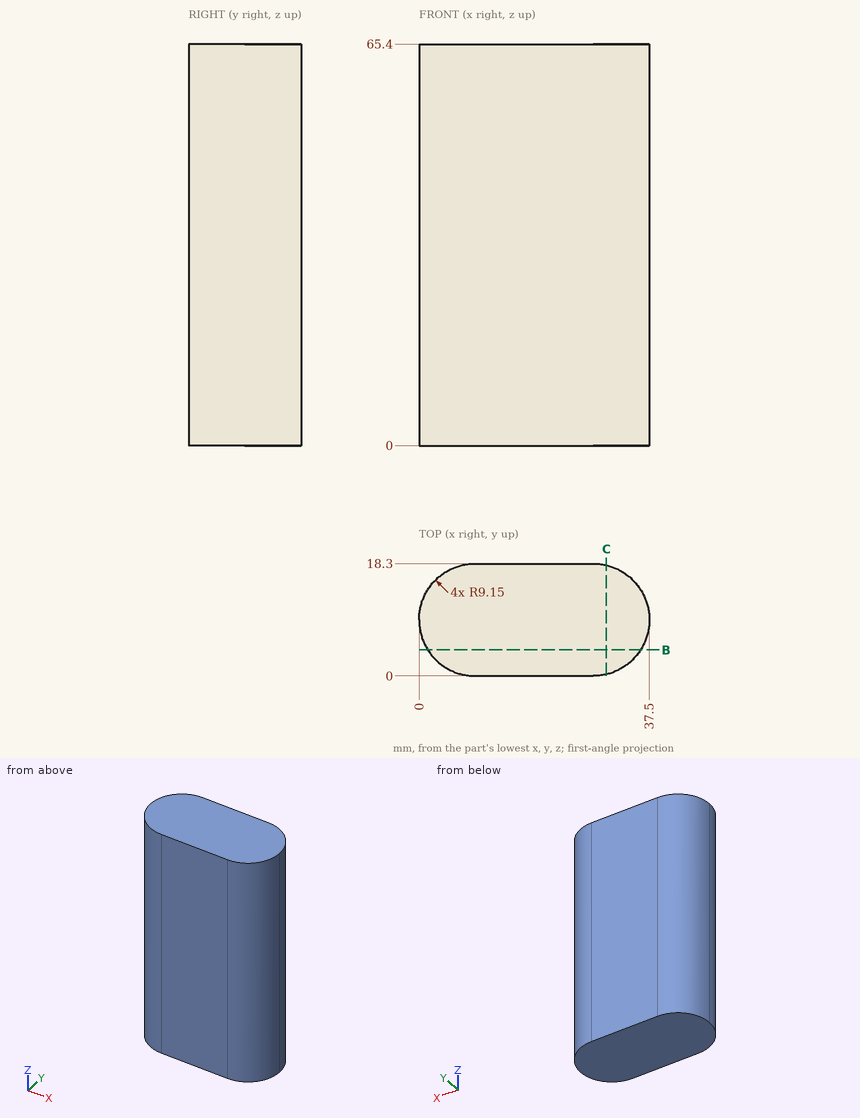
Geometry check sheet. Reference: drawing and pictorial views, mm from the part's lowest x, y, z. Give positions to 0.01 mm unless a question says otherwise; leave off trailing zeros. Write each loop counter-clockwise with the first axis right and the second up, starting at its lowest first coordinate (ties: lowest second). Pieces come first, ordered by that corner, then holes. Notation, with made-up numbers: (40, -3.5) -> (48, -3.5) arc R23 ccw to (48, 9.5) -> close; hole circle Ø6 at (51.5, -36.5). An arc over 180 degrees is marked (long way). One line per item, written item: value. Start each with the question number.
Item 1: Material ranges on probe 1 along X at (y, z) = (14.25, 5); probe 2 along X at (y, z) = (6, 36.5); probe 3 along Y at (x, z) = (7, 42.5), recorded low to high. Write a range as from..to.
Item 2: Section check B-B on y = 4.25. Record the cut outline in (x, z), then the cut area to 3 significant figures.
Item 3: Section check C-C on x = 30.5. Record the cut outline in (y, z).
Item 4: Gauge pin test, flat end, axial feed: pin 1 (10 mm diameter, centred on y = 15, z = 54.5, fed in from -X). Record the tip position at first contact, or that the pin passes through.
Results list:
1. probe 1: 1.55..35.95
1. probe 2: 0.56..36.94
1. probe 3: 0.26..18.04
2. outline: (1.42, 0) -> (36.08, 0) -> (36.08, 65.4) -> (1.42, 65.4) -> close
2. area: 2,270 mm²
3. outline: (0.26, 0) -> (18.04, 0) -> (18.04, 65.4) -> (0.26, 65.4) -> close
4. pin 1: x = 0.04
